from build123d import *

# Parameters (mm, degrees)
F0_R     = 17.5
F1_DEPTH = 100
F2_R     = 11
F3_DEPTH = 5
F4_R     = 6
F5_DEPTH = 30
F6_R     = 16
F7_DEPTH = 65
F8_W     = 5.652177
F8_H     = 10
F9_DEPTH = 55


with BuildPart() as f1:
    # F0 (on Front) → F1 (new body)
    with BuildSketch(Plane.XZ):
        Circle(F0_R)
    extrude(amount=F1_DEPTH)

    # F2 (on face) → F3 (join)
    with BuildSketch(Plane.XZ.offset(100)):
        Circle(F2_R)
    extrude(amount=F3_DEPTH)

    # F4 (on face) → F5 (cut)
    with BuildSketch(Plane.XZ.offset(105)):
        Circle(F4_R)
    extrude(amount=-F5_DEPTH, mode=Mode.SUBTRACT)

    # F6 (on Front) → F7 (join)
    with BuildSketch(Plane.XZ):
        Circle(F6_R)
    extrude(amount=-F7_DEPTH)

    # F8 (on face) → F9 (cut)
    with BuildSketch(Plane(origin=(0, 65, 0), x_dir=(-1, 0, 0), z_dir=(0, 1, 0))):
        with Locations((-18.024772, 0)):
            Rectangle(F8_W, F8_H)
    extrude(amount=-F9_DEPTH, mode=Mode.SUBTRACT)


solid = f1.part
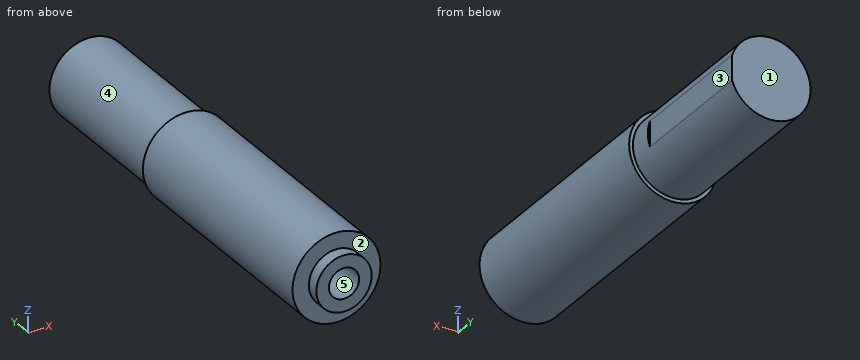
For this review, take the finished solid that the model builds, in its own axes (mm). Face numbers are marked on the shaded views. A direction names the side the tool comes from. Round coordinates to 2 decimals unless told otherwise and drop trailing zeros. Order: outer loops, then holes, each group sorted by start corner. A loop starts at its lowest first (then second) coordinate and runs counter-clockwise, first axis right, second up. Notation, with made-up numbers: M 44,65 L 59,65 A18 ccw 59,71 Z; hole C 69.25,-9 d5. An arc over 180 degrees is marked long. Write each question's results on one line, items separated by ' | '. Start each with the question number.
1. Add section B-B (z = 0). State the section outline as (x, y) points.
2. To check wall thickness, follow L1, parallel to Z at x = 0, y = -90; L2, parallel to Y at x = -14.5, z = -3.5; L3, parallel to X at y = -94.5, z = -2. State the ranges of each line that lie inside material, in increasing order. Write a range as [from, to].
3. Add section C-C (y = -77.5). State the section outline as (x, z) points.
4. Draft analysis for pull direction Z (two halves, no side actions). For the marked faces 3, 4 and 5, state which applies: pulls with the +Z half, pulls with the -Z half, needs draft (parallel to the pull), parting line crosses it, or undercut.
5. Tool access review of the marked faces 1 and 2: name each direction out of +Z, -Z, +X, -X, +Y, -Y from which nothing blocks a thin tool from reaching the whole face with its end or side.
6. Add section A-A (x = 0). State the section outline as (y, z) points.
7. Clearance check with flat-ended pins moving along their axes: pin 1 Ø5 at (x, z) = (-12.5, -6.5) entering from -Y; pin 2 Ø1 at (x, y) = (-6.5, -54.5) entering from -Z; pin 3 Ø1.5 at (x, y) = (-7, 28.5) entering from -Z. State where each tip first meets the part, or that it passes through.
8. Add section D-D (y = -9.5). State the section outline as (x, z) points, then the cut area to 3 significant figures.
Output values:
1) outline: M -17.5,-100 L -11,-100 L -11,-105 L -6,-105 L -6,-75 L 6,-75 L 6,-105 L 11,-105 L 11,-100 L 17.5,-100 L 17.5,0 L 16,0 L 16,10 L 15.2,10 L 15.2,65 L -16,65 L -16,0 L -17.5,0 Z
2) L1: [-17.5, -6], [6, 17.5] | L2: [-100, 65] | L3: [-17.39, -5.66], [5.66, 17.39]
3) outline: C 0,0 d35; hole C 0,0 d12
4) face 3: needs draft | face 4: parting line crosses it | face 5: undercut
5) face 1: +Z, -Z, +X, -X, +Y | face 2: -Y
6) outline: M -105,-11 L -100,-11 L -100,-17.5 L 0,-17.5 L 0,-16 L 65,-16 L 65,16 L 0,16 L 0,17.5 L -100,17.5 L -100,11 L -105,11 L -105,6 L -75,6 L -75,-6 L -105,-6 Z
7) pin 1: y = -100 | pin 2: z = -16.44 | pin 3: z = -14.73
8) outline: C 0,0 d35 | area: 962 mm^2
